Autodesk Inventor part; units mm, degrees
ref_plane "YZ Plane" through (0, 0, 0) normal (1, 0, 0) x (0, 1, 0)
ref_plane "XZ Plane" through (0, 0, 0) normal (0, 1, 0) x (-1, 0, 0)
ref_plane "XY Plane" through (0, 0, 0) normal (0, 0, 1) x (1, 0, 0)
sketch "Sketch1" plane through (0, 0, 0) normal (0, 1, 0) x (-1, 0, 0)
  circle A0 centre (0, 0) radius 7.5
  dimension "d0" = 15
extrude "Extrusion1" add sketch "Sketch1" along normal blind 20
sketch "Sketch2" plane through (0, 20, 0) normal (0, 1, 0) x (1, 0, 0)
  circle A0 centre (0, 0) radius 6
  dimension "d3" = 12
extrude "Extrusion2" add sketch "Sketch2" along normal blind 15
sketch "Sketch3" plane through (0, 35, 0) normal (0, 1, 0) x (1, 0, 0)
  circle A0 centre (0, 0) radius 4.5
  dimension "d6" = 9
extrude "Extrusion3" add sketch "Sketch3" along normal blind 50
sketch "Sketch4" plane through (0, 85, 0) normal (0, 1, 0) x (1, 0, 0)
  point P0 (0, 0)
fillet "Fillet1" radius 2 1 edges at (-4.5, 85, 0)
sketch "Sketch5" plane through (0, 0, 0) normal (0, -1, 0) x (1, 0, 0)
  point P0 (0, 0)
sketch "Sketch6" plane through (0, 0, 0) normal (0, -1, 0) x (1, 0, 0)
  circle A0 centre (0, 0) radius 6
  dimension "d10" = 12
extrude "Extrusion4" cut sketch "Sketch6" against normal blind 3
properties part number "Antenna that serves no purpose other than to look cool"
Geometry check sheet. Reference: the model listing, model coordinates, mm. A direction names the side the tool comes from. Coordinates: 2 decimals unless noted, no trailing zeros. Write each loop counter-clockwise with the first axis right and the second up, starting at its lowest first coordinate (ties: lowest second). Pieces come first, ordered by that corner, then holes. Notation, with made-up numbers: M -2,39 L 38,39 A23 cw 38,50 Z; hole C -29,69.5 d5. An arc over 180 degrees is marked long. Use one line per item in the form item = value. Start each with the question number.
1) Section check A-A on x = 0. Enter the section's corners in (y, z).
2) Set-up check for faces 4 (the flat face through (0, 3, 0)), 5 (the cylindrical face through (-0.59, 58.66, 4.46)), 6 (the flat face through (0, 85, 0)): record each of +Z, -Z, +X, -X, +Y, -Y from which the full face is reachable in a straight line by a thin tool's end or side.
3) Section check C-C on y = 31.5. Enter the section's corners in (x, z).
4) Section check D-D on y = 76.5. Enter the section's corners in (x, z).
5) Thickness scan on probe 1 along Z at (x, y) = (0, 0.75); probe 2 along Y at (x, z) = (-6, 1.75); probe 3 along Y at (x, z) = (-0.25, -2.5). Record the ranges inside material, lowest first. Write a range as from..to.
6) Release check for a two-part mould opening along X. For faces 1 (the cylindrical face through (7.493, 9.86, -0.33)), 2 (the cylindrical face through (-6, 1, 0)), 3 (the flat face through (-2, 20, 6)) record: pulls with the +X half, pulls with the -X half, needs draft (parallel to the pull), parting line crosses it, or undercut.
7) Go/stop test with flat-tipped pins: pin 1 Ø1.5 at (x, y) = (-2, 59.5) entering from +Z; pin 2 Ø1 at (x, z) = (-2.5, -5.5) entering from +Y; pin 3 Ø2 at (x, y) = (4, 46) entering from +Z. Record where each tip stops, or that it passes through.
8) Section check B-B on z = 0. Enter the section's corners in (x, y), and give its area (3 significant figures).
Responses:
q1.outline = M 0,-7.5 L 20,-7.5 L 20,-6 L 35,-6 L 35,-4.5 L 83,-4.5 A2 ccw 85,-2.5 L 85,2.5 A2 ccw 83,4.5 L 35,4.5 L 35,6 L 20,6 L 20,7.5 L 0,7.5 L 0,6 L 3,6 L 3,-6 L 0,-6 Z
q2.face_4 = -Y
q2.face_5 = +Y
q2.face_6 = +Z, -Z, +X, -X, +Y
q3.outline = C 0,0 d12
q4.outline = C 0,0 d9
q5.probe_1 = -7.5..-6, 6..7.5
q5.probe_2 = 0..20
q5.probe_3 = 3..85
q6.face_1 = parting line crosses it
q6.face_2 = undercut
q6.face_3 = needs draft
q7.pin_1 = 4.32
q7.pin_2 = 35
q7.pin_3 = 3.35
q8.outline = M -7.5,0 L -6,0 L -6,3 L 6,3 L 6,0 L 7.5,0 L 7.5,20 L 6,20 L 6,35 L 4.5,35 L 4.5,83 A2 ccw 2.5,85 L -2.5,85 A2 ccw -4.5,83 L -4.5,35 L -6,35 L -6,20 L -7.5,20 Z
q8.area = 892 mm2
